```python
from build123d import *

# Parameters (mm, degrees)
SKETCH1_R      = 3
EXTRUDE1_DEPTH = 2
SKETCH2_R      = 0.75
EXTRUDE2_DEPTH = 2


with BuildPart() as part:
    # Sketch1 → Extrude1 (new body)
    with BuildSketch(Plane.XY):
        with BuildLine():
            Line((13.471864542, 10.121208711), (4.054216685, -2.926316298))
            ThreePointArc((4.054216685, -2.926316298), (0, -5), (-4.054216685, -2.926316298))
            Line((-4.054216685, -2.926316298), (-13.471864542, 10.121208711))
            ThreePointArc((-13.471864542, 10.121208711), (-13.190330714, 13.254849624), (-10.048252993, 13.417066342))
            Line((-10.048252993, 13.417066342), (-1.231322951, 6.52852563))
            ThreePointArc((-1.231322951, 6.52852563), (0, 6.104547138), (1.231322951, 6.52852563))
            Line((1.231322951, 6.52852563), (10.048252993, 13.417066342))
            ThreePointArc((10.048252993, 13.417066342), (13.190330714, 13.254849624), (13.471864542, 10.121208711))
        make_face()
        Circle(SKETCH1_R, mode=Mode.SUBTRACT)
    extrude(amount=EXTRUDE1_DEPTH)

    # Sketch2 → Extrude2 (cut)
    with BuildSketch(Plane.XY.offset(2)):
        with Locations((11.525840533, 11.525840533)):
            Circle(SKETCH2_R)
        with Locations((9.40452019, 9.40452019)):
            Circle(SKETCH2_R)
        with Locations((7.283199846, 7.283199846)):
            Circle(SKETCH2_R)
        with Locations((5.161879503, 5.161879503)):
            Circle(SKETCH2_R)
        with Locations(Location((-5.161879503, 5.161879503, 0), (0, 0, 180))):
            Circle(SKETCH2_R)
        with Locations(Location((-7.283199846, 7.283199846, 0), (0, 0, 180))):
            Circle(SKETCH2_R)
        with Locations(Location((-9.40452019, 9.40452019, 0), (0, 0, 180))):
            Circle(SKETCH2_R)
        with Locations(Location((-11.525840533, 11.525840533, 0), (0, 0, 180))):
            Circle(SKETCH2_R)
    extrude(amount=-EXTRUDE2_DEPTH, mode=Mode.SUBTRACT)


solid = part.part
```
Read the model definition and answer for the solid it produces. Units are mm, in the model's axes. A direction names the side the tool comes from. Give positions to 0.01 mm unless a question says otherwise; leave off trailing zeros. Write each loop counter-clockwise with the first axis right and the second up, starting at its lowest first coordinate (ties: lowest second). Pieces come first, ordered by that corner, then holes. Notation, with made-up numbers: M 18,43 L 60,43 A22 cw 60,54 Z; hole C -35,3.5 d1. An arc over 180 degrees is marked long. Put each result on its own line as item: value. Start each with the question number.
1. For a pull along X with two mould halves and no side action, classify faces 1 (the cylindrical face through (-0.019, 6.105, 0.986)), 2 (the cylindrical face through (0, -5, 1)), 3 (the cylindrical face through (13.155, 13.288, 0.986)), 4 (the flat face through (8.83, 3.69, 0.99)) as released by +X, released by -X, zero draft, split by the parting line, or undercut.
2. The part is cut by section C-C, the plane z = 0.6. Give the number of separate pieces and of enclosed holes in the cut face, and give its area (3 significant figures).
3. Consider line 1 along X through (y, z) = (7.5, 0.4); line 2 along X through (y, z) = (12, 0.75); line 3 along Y through (x, z) = (0, 0.9). Determine where each line is inside the solid, lowest interval first.
4. This flat-tipped pin is pushed along its axis until it touches: pin 1 Ø1.7 at (x, y) = (-9.4, 9.4) entering from -Z. Where does it stop, or does it pass through?
5. Which of the six approach directions +Z, -Z, +X, -X, +Y, -Y give full straight-line access (tool end or side, diameter ignored) to faces 5 (the cylindrical face through (-13.225, 13.221, 0.986)), 6 (the flat face through (-5.7, 10.02, 0.99))?
6. The part is cut by section A-A, the plane x = 0. Give the vertices of the cut face in (y, z), and give its area (3 significant figures).
7. The part is cut by section B-B, the plane y = 0. Give the vertices of the cut face in (x, z).
Final values:
1. face 1: undercut
1. face 2: split by the parting line
1. face 3: undercut
1. face 4: released by +X
2. separate pieces: 1
2. enclosed holes: 9
2. area: 212 mm²
3. line 1: x = -11.58 to -8, -6.57 to -2.47, 2.47 to 6.57, 8 to 11.58
3. line 2: x = -13.88 to -12.11, -10.94 to -8.23, 8.23 to 10.94, 12.11 to 13.88
3. line 3: y = -5 to -3, 3 to 6.1
4. pin 1: stops at z = 0
5. face 5: +Z, -Z
5. face 6: +Z, -Z, +Y
6. outline: M -5,0 L -3,0 L -3,2 L -5,2 Z; M 3,0 L 6.1,0 L 6.1,2 L 3,2 Z
6. area: 10.2 mm²
7. outline: M -6.17,0 L -3,0 L -3,2 L -6.17,2 Z; M 3,0 L 6.17,0 L 6.17,2 L 3,2 Z
